from build123d import *

# Parameters (mm, degrees)
SZKIC1_R                    = 22.5
DODANIE_WYCI_GNI_CIE2_DEPTH = 13
SZKIC2_W                    = 220
SZKIC2_H                    = 30
DODANIE_WYCI_GNI_CIE3_DEPTH = 6
ZAOKR_GLENIE1_R             = 10
SZKIC4_R                    = 20.5
WYTNIJ_WYCI_GNI_CIE3_DEPTH  = 11
WYTNIJ_WYCI_GNI_CIE2_DEPTH  = 4
WYTNIJ_WYCI_GNI_CIE4_REACH  = 173.975
SZKIC8_W                    = 23
SZKIC8_H                    = 14
SZKIC12_R                   = 3.3
DODANIE_WYCI_GNI_CIE4_DEPTH = 3
OTW_R_POD_RUB_M21_D         = 2.6
OTW_R_POD_RUB_M23_D         = 2.6
SZKIC14_R                   = 3.3
DODANIE_WYCI_GNI_CIE5_DEPTH = 5
OTW_R_POD_RUB_M24_D         = 2.6
SZKIC15_W                   = 6
SZKIC15_H                   = 6
SZKIC15_W_2                 = 4
SZKIC15_H_2                 = 4
DODANIE_WYCI_GNI_CIE6_DEPTH = 10
SZYK_LINIOWY1_COUNT         = 2
SZYK_LINIOWY1_PITCH         = 70
OTW_R_POD_RUB_M25_D         = 2.4


with BuildPart() as part:
    # Szkic1 → Dodanie-wyciągnięcie2 (new body)
    with BuildSketch(Plane.XY):
        with Locations(Location((0, 0, 0), (0, 0, 180))):
            Circle(SZKIC1_R)
    extrude(amount=DODANIE_WYCI_GNI_CIE2_DEPTH)

    # Szkic2 → Dodanie-wyciągnięcie3 (add)
    with BuildSketch(Plane.XY):
        with Locations((60, 0)):
            Rectangle(SZKIC2_W, SZKIC2_H)
    extrude(amount=DODANIE_WYCI_GNI_CIE3_DEPTH)

    # Zaokrąglenie1
    zaokr_glenie1_edges = [part.edges().sort_by_distance(p)[0] for p in [
        (170, 15, 3),
        (-50, -15, 3),
        (170, -15, 3),
        (-50, 15, 3),
    ]]
    fillet(zaokr_glenie1_edges, radius=ZAOKR_GLENIE1_R)

    # Szkic4 → Wytnij-wyciągnięcie3 (cut)
    with BuildSketch(Plane.XY.offset(13)):
        Circle(SZKIC4_R)
    extrude(amount=-WYTNIJ_WYCI_GNI_CIE3_DEPTH, mode=Mode.SUBTRACT)

    # Szkic3 → Wytnij-wyciągnięcie2 (cut)
    with BuildSketch(Plane.XY.offset(6)):
        with BuildLine():
            Line((168, -5), (168, 5))
            ThreePointArc((168, 5), (165.656854249, 10.656854249), (160, 13))
            Line((160, 13), (20.766559657, 13))
            ThreePointArc((20.766559657, 13), (24.5, 0), (20.766559657, -13))
            Line((20.766559657, -13), (160, -13))
            ThreePointArc((160, -13), (165.656854249, -10.656854249), (168, -5))
        make_face()
        with BuildLine():
            Line((-48, 5), (-48, -5))
            ThreePointArc((-48, -5), (-45.656854249, -10.656854249), (-40, -13))
            Line((-40, -13), (-20.766559657, -13))
            ThreePointArc((-20.766559657, -13), (-24.5, 0), (-20.766559657, 13))
            Line((-20.766559657, 13), (-40, 13))
            ThreePointArc((-40, 13), (-45.656854249, 10.656854249), (-48, 5))
        make_face()
    extrude(amount=-WYTNIJ_WYCI_GNI_CIE2_DEPTH, mode=Mode.SUBTRACT)

    # Szkic8 → Wytnij-wyciągnięcie4 (cut, up to next)
    with BuildSketch(Plane.XY, mode=Mode.PRIVATE) as wytnij_wyci_gni_cie4_sk1:
        with Locations((150, 0)):
            Rectangle(SZKIC8_W, SZKIC8_H)
    wytnij_wyci_gni_cie4_tool1 = extrude(wytnij_wyci_gni_cie4_sk1.sketch, amount=WYTNIJ_WYCI_GNI_CIE4_REACH, mode=Mode.PRIVATE) & part.part
    add(wytnij_wyci_gni_cie4_tool1.solids().sort_by_distance((150, 0, 0))[0], mode=Mode.SUBTRACT)

    # Szkic12 → Dodanie-wyciągnięcie4 (add)
    with BuildSketch(Plane.XY.offset(2)):
        Circle(SZKIC12_R)
    extrude(amount=DODANIE_WYCI_GNI_CIE4_DEPTH)

    # Otwór pod śrubę M21 (through all)
    with Locations(Plane(origin=(0, 0, 0), x_dir=(1, 0, 0), z_dir=(0, 0, -1))):
        with Locations((0, 0)):
            Hole(OTW_R_POD_RUB_M21_D / 2)

    # Otwór pod śrubę M23 (through all)
    with Locations(Plane(origin=(0, 0, 0), x_dir=(1, 0, 0), z_dir=(0, 0, -1))):
        with Locations((136, 0), (164, 0)):
            Hole(OTW_R_POD_RUB_M23_D / 2)

    # Szkic14 → Dodanie-wyciągnięcie5 (add)
    with BuildSketch(Plane.XY.offset(2)):
        with Locations((-40, 0)):
            Circle(SZKIC14_R)
    extrude(amount=DODANIE_WYCI_GNI_CIE5_DEPTH)

    # Otwór pod śrubę M24 (through all)
    with Locations(Plane(origin=(-40, 0, 0), x_dir=(-1, 0, 0), z_dir=(0, 0, -1))):
        with Locations((0, 0)):
            Hole(OTW_R_POD_RUB_M24_D / 2)

    # Szkic15 → Dodanie-wyciągnięcie6 (add)
    with BuildSketch(Plane(origin=(130, 0, 0), x_dir=(0, 0, -1), z_dir=(1, 0, 0))):
        with Locations((-3, 18)):
            Rectangle(SZKIC15_W, SZKIC15_H)
        with Locations((-3, 18)):
            Rectangle(SZKIC15_W_2, SZKIC15_H_2, mode=Mode.SUBTRACT)
    dodanie_wyci_gni_cie6 = extrude(amount=-DODANIE_WYCI_GNI_CIE6_DEPTH)

    # Szyk liniowy1: Dodanie-wyciągnięcie6 ×2
    with Locations(*[(-i * SZYK_LINIOWY1_PITCH, 0, 0) for i in range(1, SZYK_LINIOWY1_COUNT)]):
        add(dodanie_wyci_gni_cie6)

    # Otwór pod śrubę M25 (through all)
    with Locations(Plane.XY.offset(2)):
        with Locations((55, -10), (105, -10), (105, 10), (55, 10)):
            Hole(OTW_R_POD_RUB_M25_D / 2)

    # Cięcie powierzchnią1
    split(bisect_by=Plane(origin=(80, 0, 0), x_dir=(0, 0, -1), z_dir=(1, 0, 0)), keep=Keep.BOTTOM)


solid = part.part
Geometry check sheet. Reference: the model listing, model coordinates, mm. A direction names the side the tool comes from. Give positions to 0.01 mm unless a question says otherwise; leave off trailing zeros. Order: outer loops, then holes, each group sorted by start corner. A loop starts at its lowest first (then second) coordinate and runs counter-clockwise, first axis right, second up. Notation, with made-up numbers: (87.5, -34) - (145.5, -34) arc R13 cw to (145.5, -29) - close; hole circle Ø9 at (-12, 53.5). An arc over 180 degrees is marked (long way). Use one line per item in the form item = value.
1) Sectioned sample at B-B (y = 0). Count the separate pieces of the cut face and the enclosed holes in it, and give its area (3 significant figures).
Working result:
separate_pieces = 3
enclosed_holes = 0
area = 350 mm^2
2) Sectioned sample at D-D (x = 70). Record the boundary of the cut face in (y, z), and give its area (3 significant figures).
Working result:
outline = (-15, 0) - (15, 0) - (15, 6) - (13, 6) - (13, 2) - (-13, 2) - (-13, 6) - (-15, 6) - close
area = 76.0 mm^2
3) Sectioned sample at C-C (y = 10). Record the boundary of the cut face in (x, z) (3 decimals), and give its area (3 significant figures).
Working result:
outline = (-48.66, 0) - (53.8, 0) - (53.8, 2) - (22.366, 2) - (22.366, 6) - (20.156, 6) - (20.156, 13) - (17.896, 13) - (17.896, 2) - (-17.896, 2) - (-17.896, 13) - (-20.156, 13) - (-20.156, 6) - (-22.366, 6) - (-22.366, 2) - (-46.245, 2) - (-46.245, 6) - (-48.66, 6) - close; (56.2, 0) - (80, 0) - (80, 2) - (56.2, 2) - close
area = 330 mm^2
4) Sectioned sample at A-A (x = 55). Record the boundary of the cut face in (y, z), and give its area (3 significant figures).
Working result:
outline = (-15, 0) - (-11.2, 0) - (-11.2, 2) - (-13, 2) - (-13, 6) - (-15, 6) - close; (-8.8, 0) - (8.8, 0) - (8.8, 2) - (-8.8, 2) - close; (11.2, 0) - (21, 0) - (21, 6) - (13, 6) - (13, 2) - (11.2, 2) - close; hole (16, 1) - (20, 1) - (20, 5) - (16, 5) - close
area = 86.4 mm^2
5) Access from +Z, -Z, +X, -X, +Y, -Y to the whole of each face (thin tool, end or side, straight path). Record for faces 1 (the face through (-2.43, 2.23, 3.48)), 2 (the face through (70, 15, 3)), 3 (the face through (-29, 15, 3)).
Working result:
face_1 = +Z
face_2 = +Z, -Z, +X, +Y
face_3 = +Z, -Z, -X, +Y
6) Draft check along Z on faces 4 (the face through (55, 18, 1)), 5 (the face through (14, 0, 0)), 6 (the face through (-48, 0, 4)). Enter one of: released by +Z, released by -Z, zero draft, split by the parting line, or undercut.
Working result:
face_4 = undercut
face_5 = released by -Z
face_6 = zero draft
7) Material ranges on probe 1 along Y at (x, z) = (55, 1.05); probe 2 along Z at (x, y) = (59, 17); probe 3 along Y at (x, z) = (-2, 4.75), recorded low to high. Write a range as from..to.
Working result:
probe_1 = -15..-11.2, -8.8..8.8, 11.2..16, 20..21
probe_2 = 0..1, 5..6
probe_3 = -22.41..-20.4, -2.62..2.62, 20.4..22.41
8) Depth check by flat-ended pin: pin 1 Ø3 at (x, z) = (39, 3) entering from +Y; pin 2 Ø5 at (y, z) = (-14, 9) entering from +X; pin 3 Ø3 at (x, z) = (-28, 4) entering from -Y. Enter the tip coordinate at first touch or a pass-through.
Working result:
pin_1 = 15
pin_2 = 19.34
pin_3 = -15
